```python
from build123d import *

# Parameters (mm, degrees)
BOSS_EXTRUDE9_DEPTH  = 5
SKETCH6_3_R          = 2
BOSS_EXTRUDE10_DEPTH = 10


with BuildPart() as part:
    # Sketch6 → Boss-Extrude9 (new body)
    with BuildSketch(Plane(origin=(0, 0, 0), x_dir=(1, 0, 0), z_dir=(0, 1, 0))):
        Polygon((98.912801806, 26.664335605), (8.912801806, 26.664335605), (8.912801806, -18.335664395), (43.912801806, -18.335664395), (43.912801806, -3.335664395), (83.912801806, -3.335664395), (83.912801806, -18.335664395), (98.912801806, -18.335664395), align=None)
    extrude(amount=BOSS_EXTRUDE9_DEPTH)

    # Sketch6_3 → Boss-Extrude10 (add)
    with BuildSketch(Plane(origin=(0, 0, 0), x_dir=(1, 0, 0), z_dir=(0, 1, 0))):
        with Locations(Location((13.412801806, 22.164335605, 0), (0, 0, 270))):
            Circle(SKETCH6_3_R)
        with Locations(Location((93.912801806, 21.664335605, 0), (0, 0, 270))):
            Circle(SKETCH6_3_R)
        with Locations(Location((93.912801806, -13.835664395, 0), (0, 0, 270))):
            Circle(SKETCH6_3_R)
        with Locations(Location((13.412801806, -13.835664395, 0), (0, 0, 270))):
            Circle(SKETCH6_3_R)
    extrude(amount=BOSS_EXTRUDE10_DEPTH)


solid = part.part
```
Verification items for the finished model (mm, model axes). A direction names the side the tool comes from. Round coordinates to 2 decimals unless told otherwise and drop trailing zeros. Order: outer loops, then holes, each group sorted by start corner. A loop starts at its lowest first (then second) coordinate and runs counter-clockwise, first axis right, second up. Notation, with made-up numbers: (-7, -2.5) - (14, -2.5) arc R9 cw to (14, 3.5) - close; hole circle Ø9 at (43.5, 43). An arc over 180 degrees is marked (long way). Use CSV: the item, a comma, the result in double quotes. Start each with the question number.
1) Mould release check, pull along Z, two halves, no side actions. Record for faces 4 (the flat face through (13, 10, 14)), 5 (the flat face through (26, 2, 18.336)), 6 (the cylindrical face through (95.9, 7.5, 13.6)): +Z half, -Z half, draft (parallel to the pull), parting line (faces both ways), or undercut.
2) Section check A-A, the plane z = 15. Record the cut outline in (x, y), plus the area to 3 significant figures.
3) Go/stop test with flat-tipped pins: P1, Ø12, axis at x = 34, z = 5, coming from the +Y side; P2, Ø1.5, axis at x = 69, y = 2, coming from the +Z side. Record where each tip stops, or that it passes through.
4) Section check D-D, the plane y = 7.25. Record the cut outline in (x, z), plus the area to 3 significant figures.
5) Access from +Z, -Z, +X, -X, +Y, -Y to the whole of each face (thin tool, end or side, straight path). Record for faces 1 (the flat face through (83.913, 2, 11)), 2 (the cylindrical face through (15.4, 7.5, 13.6)), 3 (the flat face through (8.913, 2, -4)).
6) Section check C-C, the plane x = 47.5. Record the cut outline in (y, z).
7) Section check B-B, the plane y = 2.5. Record the cut outline in (x, z), plus the area to 3 significant figures.
8) Thickness scan on L1, parallel to X at y = 1.5, z = 7.5; L2, parallel to Y at x = 24.5, z = 9; L3, parallel to X at y = 9.5, z = 15. Record the ranges inside material, lowest first.
Answers:
1,face 4,"draft"
1,face 5,"+Z half"
1,face 6,"undercut"
2,outline,"(8.91, 0) - (43.91, 0) - (43.91, 5) - (15.04, 5) - (15.04, 10) - (11.79, 10) - (11.79, 5) - (8.91, 5) - close; (83.91, 0) - (98.91, 0) - (98.91, 5) - (95.54, 5) - (95.54, 10) - (92.29, 10) - (92.29, 5) - (83.91, 5) - close"
2,area,"283 mm²"
3,P1,"stops at y = 5"
3,P2,"stops at z = 3.34"
4,outline,"circle Ø4 at (13.41, -22.16); circle Ø4 at (13.41, 13.84); circle Ø4 at (93.91, -21.66); circle Ø4 at (93.91, 13.84)"
4,area,"50.3 mm²"
5,face 1,"+Z, +Y, -Y"
5,face 2,"+Y"
5,face 3,"+Z, -Z, -X, +Y, -Y"
6,outline,"(0, -26.66) - (5, -26.66) - (5, 3.34) - (0, 3.34) - close"
7,outline,"(8.91, -26.66) - (98.91, -26.66) - (98.91, 18.34) - (83.91, 18.34) - (83.91, 3.34) - (43.91, 3.34) - (43.91, 18.34) - (8.91, 18.34) - close"
7,area,"3,450 mm²"
8,L1,"x = 8.91 to 43.91, 83.91 to 98.91"
8,L2,"y = 0 to 5"
8,L3,"x = 11.79 to 15.04, 92.29 to 95.54"
